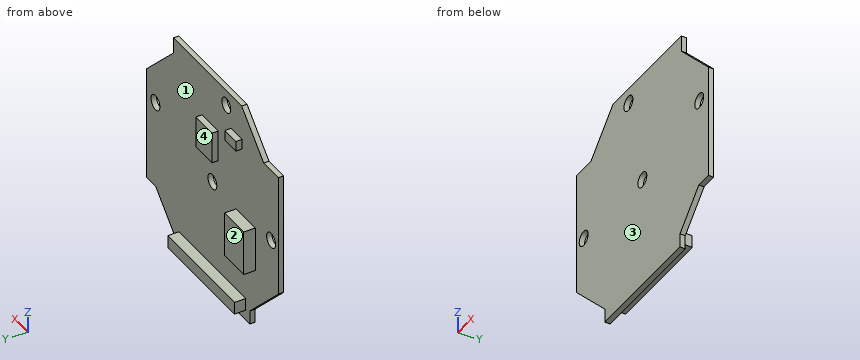
from build123d import *

# Parameters (mm, degrees)
BOSS_EXTRUDE1_DEPTH = 0.85
SKETCH2_W           = 18.2
SKETCH2_H           = 2
BOSS_EXTRUDE2_DEPTH = 1.8
SKETCH3_W           = 5.2
SKETCH3_H           = 7.3
BOSS_EXTRUDE3_DEPTH = 1.88
SKETCH4_W           = 4.4
SKETCH4_H           = 5.1
SKETCH4_W_2         = 3
SKETCH4_H_2         = 1.65
BOSS_EXTRUDE4_DEPTH = 1
SKETCH5_R           = 1.21
CUT_EXTRUDE1_DEPTH  = 1.85


with BuildPart() as part:
    # Sketch1 → Boss-Extrude1 (new body)
    with BuildSketch(Plane(origin=(0, 0, 0), x_dir=(1, 0, 0), z_dir=(0, 1, 0))):
        Polygon((-10.25, 18), (10.25, 18), (10.25, 15.75), (15.4, 10.6), (18, 10.6), (18, -8), (10.6, -15.4), (10.6, -18), (-8, -18), (-14, -12), (-18, -12), (-18, 8), (-10.25, 15.75), align=None)
    extrude(amount=BOSS_EXTRUDE1_DEPTH)

    # Sketch2 → Boss-Extrude2 (add)
    with BuildSketch(Plane(origin=(0, 0.85, 0), x_dir=(1, 0, 0), z_dir=(0, 1, 0))):
        with Locations((0, 15.35)):
            Rectangle(SKETCH2_W, SKETCH2_H)
    extrude(amount=BOSS_EXTRUDE2_DEPTH)

    # Sketch3 → Boss-Extrude3 (add)
    with BuildSketch(Plane(origin=(0, 0.85, 0), x_dir=(1, 0, 0), z_dir=(0, 1, 0))):
        with Locations((-9.1, 4.25)):
            Rectangle(SKETCH3_W, SKETCH3_H)
    extrude(amount=BOSS_EXTRUDE3_DEPTH)

    # Sketch4 → Boss-Extrude4 (add)
    with BuildSketch(Plane(origin=(0, 0.85, 0), x_dir=(1, 0, 0), z_dir=(0, 1, 0))):
        with Locations((0.6, -7.15)):
            Rectangle(SKETCH4_W, SKETCH4_H)
        with Locations((-6.6, -11.525)):
            Rectangle(SKETCH4_W_2, SKETCH4_H_2)
    extrude(amount=BOSS_EXTRUDE4_DEPTH)

    # Sketch5 → Cut-Extrude1 (cut, through all)
    with BuildSketch(Plane(origin=(0, 0.85, 0), x_dir=(1, 0, 0), z_dir=(0, 1, 0))):
        Circle(SKETCH5_R)
        with Locations((-16, 0)):
            Circle(SKETCH5_R)
        with Locations((-3.8, -15.5)):
            Circle(SKETCH5_R)
        with Locations((15.5, -3.8)):
            Circle(SKETCH5_R)
    extrude(amount=-CUT_EXTRUDE1_DEPTH, mode=Mode.SUBTRACT)


solid = part.part
The listing builds one solid part. Answer for the finished solid, in the listing's coordinates (mm). Face numbers are marked on the shaded views. A direction names the side the tool comes from. Give positions to 0.01 mm unless a question says otherwise; leave off trailing zeros. Write each loop counter-clockwise with the first axis right and the second up, starting at its lowest first coordinate (ties: lowest second). Pieces come first, ordered by that corner, then holes.
1) Given P1, Ø4, axis at x = -16, z = 0, coming from the -Y side; P2, Ø1.4, axis at x = 2.5, y = 2, coming from the -Z side; P3, Ø2, axis at x = 1.5, z = -15.5, coming from the +Y side; P4, Ø0.5, axis at x = 0, y = 1.5, coming from the +Z side, each flat-ended and moving along its own axis, determine where each tip first touches the part or whether it passes through.
2) Section C-C (z = 3.8) is taken. Write down the section's boundary in (x, y), and give its area (3 significant figures).
3) Section B-B (x = -16) is taken. Write down the section's boundary in (y, z), and give its area (3 significant figures).
4) For a pull along Z with two mould halves and no side action, classify the marked faces 1 and 2 as pulls with the +Z half, pulls with the -Z half, needs draft (parallel to the pull), parting line crosses it, or undercut.
5) Section A-A (z = 0) is taken. Write down the section's boundary in (x, y), and give its area (3 significant figures).
6) Find the intervals of material crossed by L1, parallel to X at y = 0.5, z = 0; L2, parallel to X at y = 0.5, z = 3.8, in increasing order.
7) Section D-D (z = -15) is taken. Write down the section's boundary in (x, y).
8) A tool of negligible diameter and unlimited length cuts with its end or side. For the marked faces 3 and 4, from which of +Z, -Z, +X, -X, +Y, -Y can it reach the whole face along a straight path? Write none if from no direction.
Response:
1. P1: stops at y = 0
1. P2: stops at z = -16.35
1. P3: stops at y = 2.65
1. P4: stops at z = 9.7
2. outline: (-18, 0) - (14.29, 0) - (14.29, 0.85) - (-18, 0.85) - close; (16.71, 0) - (18, 0) - (18, 0.85) - (16.71, 0.85) - close
2. area: 28.5 mm2
3. outline: (0, -10) - (0.85, -10) - (0.85, -1.21) - (0, -1.21) - close; (0, 1.21) - (0.85, 1.21) - (0.85, 12) - (0, 12) - close
3. area: 16.6 mm2
4. face 1: undercut
4. face 2: needs draft
5. outline: (-18, 0) - (-17.21, 0) - (-17.21, 0.85) - (-18, 0.85) - close; (-14.79, 0) - (-1.21, 0) - (-1.21, 0.85) - (-14.79, 0.85) - close; (1.21, 0) - (18, 0) - (18, 0.85) - (1.21, 0.85) - close
5. area: 26.5 mm2
6. L1: x = -18 to -17.21, -14.79 to -1.21, 1.21 to 18
6. L2: x = -18 to 14.29, 16.71 to 18
7. outline: (-11, 0) - (11, 0) - (11, 0.85) - (9.1, 0.85) - (9.1, 2.65) - (-9.1, 2.65) - (-9.1, 0.85) - (-11, 0.85) - close
8. face 3: +Z, -Z, +X, -X, -Y
8. face 4: +Z, +X, -X, +Y
